The listing builds one solid part. Answer for the finished solid, in the listing's coordinates (mm). Face numbers are marked on the shaded views. A direction names the side the tool comes from. Give positions to 0.01 mm unless a question says otherwise; leave off trailing zeros. Write each loop counter-clockwise with the first axis right and the second up, starting at its lowest first coordinate (ties: lowest second). Pieces come first, ordered by that corner, then holes.
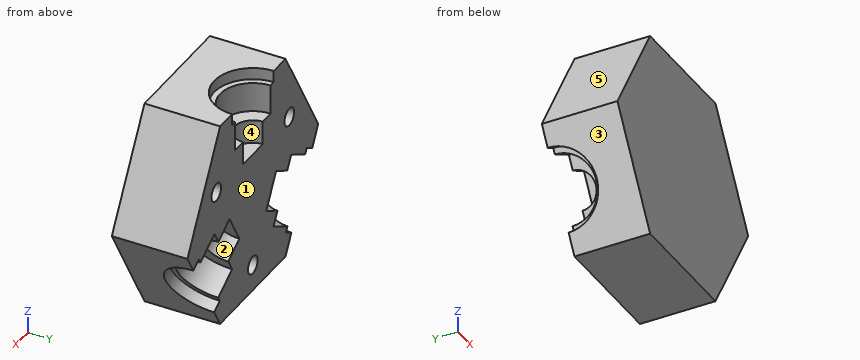
```python
from build123d import *

# Parameters (mm, degrees)
BOSS_EXTRUDE1_DEPTH = 12.7
CIRPATTERN1_COUNT   = 3
SKETCH7_R           = 1.5
CUT_EXTRUDE2_DEPTH  = 6.35


with BuildPart() as part:
    # Sketch1 → Boss-Extrude1 (new body)
    with BuildSketch(Plane(origin=(0, 0, 0), x_dir=(1, 0, 0), z_dir=(0, 1, 0))):
        Polygon((10.16, -17.597636205), (20.32, 0), (10.16, 17.597636205), (-10.16, 17.597636205), (-20.32, 0), (-10.16, -17.597636205), align=None)
    extrude(amount=BOSS_EXTRUDE1_DEPTH)

    # Sketch5 → Cut-Revolve1 (revolve, cut)
    with BuildSketch(Plane(origin=(0, 12.7, 0), x_dir=(1, 0, 0), z_dir=(0, 1, 0))):
        Polygon((0, -17.597636205), (0, -6.597636205), (-3.065310501, -6.597636205), (-3.065310501, -10.597636205), (-5.5, -10.597636205), (-5.5, -15.597636205), (-6.5, -15.597636205), (-6.5, -17.597636205), align=None)
    cut_revolve1 = revolve(axis=Axis((0, 12.7, 17.597636205), (0, 0, -1)), mode=Mode.SUBTRACT)

    # CirPattern1: Cut-Revolve1 ×3 about axis
    cirpattern1_axis = Axis((0, 0, 0), (0, 1, 0))
    for i in range(1, CIRPATTERN1_COUNT):
        add(cut_revolve1.rotate(cirpattern1_axis, i * 360 / CIRPATTERN1_COUNT), mode=Mode.SUBTRACT)

    # Sketch7 → Cut-Extrude2 (cut)
    with BuildSketch(Plane(origin=(0, 12.7, 0), x_dir=(1, 0, 0), z_dir=(0, 1, 0))):
        with Locations((0, 13.097636205)):
            Circle(SKETCH7_R)
        with Locations((11.342885683, -6.548818102)):
            Circle(SKETCH7_R)
        with Locations((-11.342885683, -6.548818102)):
            Circle(SKETCH7_R)
    extrude(amount=-CUT_EXTRUDE2_DEPTH, mode=Mode.SUBTRACT)


solid = part.part
```
Item 1: Consider probe 1 along X at (y, z) = (12, -1.5); probe 2 along X at (y, z) = (11.5, -1.5); probe 3 along Z at (x, y) = (0, 9.25). Determine where each line is inside the solid, lowest interval first.
Conclusion:
probe 1: x = -19.45 to -13.51, -11.37 to -8.57, -6.75 to 6.75, 8.57 to 11.37, 13.51 to 19.45
probe 2: x = -19.45 to -13.33, -11.37 to -8.24, -6.75 to 6.75, 8.24 to 11.37, 13.33 to 19.45
probe 3: z = -17.6 to -14.6, -11.6 to 10.6
Item 2: Each of these flat-tipped pins is pushed along its axis until it touches: P1, Ø2.5, axis at x = 0.5, z = -13, coming from the +Y side; P2, Ø1, axis at x = 13, y = 9, coming from the +Z side; P3, Ø6, axis at y = 6, z = 10, coming from the -X side; P4, Ø2, axis at x = -1.5, y = 10, coming from the +Z side. Where does it stop, or does it pass through?
Conclusion:
P1: stops at y = 12.7
P2: stops at z = 13.54
P3: stops at x = -16.28
P4: stops at z = 10.6
Item 3: A cutting plane is placed at A-A, the plane x = 0. Give the vertices of the cut face in (y, z).
Conclusion:
outline: (0, -17.6) - (12.7, -17.6) - (12.7, -14.6) - (6.35, -14.6) - (6.35, -11.6) - (12.7, -11.6) - (12.7, 6.6) - (9.63, 6.6) - (9.63, 10.6) - (7.2, 10.6) - (7.2, 15.6) - (6.2, 15.6) - (6.2, 17.6) - (0, 17.6) - close
Item 4: A cutting plane is placed at B-B, the plane y = 1.25. Give the vertices of the cut face in (x, z).
Conclusion:
outline: (-20.32, 0) - (-10.16, -17.6) - (10.16, -17.6) - (20.32, 0) - (10.16, 17.6) - (-10.16, 17.6) - close
Item 5: A cutting plane is placed at C-C, the plane y = 11. Count the separate pieces of the cut face and the enclosed holes in it, plus the area to 3 significant figures.
Conclusion:
separate pieces: 1
enclosed holes: 3
area: 758 mm2
Item 6: A cutting plane is placed at D-D, the plane z = 4.5. Give the vertices of the cut face in (x, y), plus the area to 3 significant figures.
Conclusion:
outline: (-17.72, 0) - (17.72, 0) - (17.72, 12.7) - (-17.72, 12.7) - close
area: 450 mm2
Item 7: Determine the mould class of the marked faces 1, 2 and 3 for opening direction X: pulls with the +X half, pulls with the -X half, needs draft (parallel to the pull), parting line crosses it, or undercut.
Conclusion:
face 1: needs draft
face 2: undercut
face 3: pulls with the -X half
Item 8: Which of the six approach directions +Z, -Z, +X, -X, +Y, -Y give full straight-line access (tool end or side, diameter ignored) to the marked faces 4 and 5?
Conclusion:
face 4: +Z, +Y
face 5: +Z, -X, +Y, -Y
